```python
from build123d import *

# Parameters (mm, degrees)
BASE_W                 = 11.6
BASE_H                 = 22.8
MAIN_DEPTH             = 5
GEAR_AXIS_HOLES_D      = 5
M2_5_CLEARANCE_HOLE1_D = 2.9
FILLET1_R              = 3
FILLET2_R              = 1.5


with BuildPart() as part:
    # Base → Main (new body)
    with BuildSketch(Plane.XY):
        Polygon((0, 27.5), (-26.7, 27.5), (-26.7, -27.5), (0, -27.5), (0, -39.47), (26.6, -39.47), (31.6, -39.47), (31.6, 27.5), (26.6, 27.5), align=None)
        with Locations((13.3, -14.97)):
            Rectangle(BASE_W, BASE_H, mode=Mode.SUBTRACT)
    extrude(amount=MAIN_DEPTH)

    # Gear Axis Holes (through all)
    with Locations(Plane(origin=(0, 0, 0), x_dir=(-1, 0, 0), z_dir=(0, 0, -1))):
        with Locations((16.7, -20), (16.7, 20)):
            Hole(GEAR_AXIS_HOLES_D / 2)

    # M2.5 Clearance Hole1 (through all)
    with Locations(Plane.XY.offset(5)):
        with Locations((13.3, -0.47), (13.3, -29.47)):
            Hole(M2_5_CLEARANCE_HOLE1_D / 2)

    # Fillet1
    fillet1_edges = [part.edges().sort_by_distance(p)[0] for p in [
        (31.6, 27.5, 2.5),
        (31.6, -39.47, 2.5),
        (0, -39.47, 2.5),
        (0, -27.5, 2.5),
        (-26.7, -27.5, 2.5),
        (-26.7, 27.5, 2.5),
    ]]
    fillet(fillet1_edges, radius=FILLET1_R)

    # Fillet2
    fillet2_edges = [part.edges().sort_by_distance(p)[0] for p in [
        (19.1, -26.37, 2.5),
        (19.1, -3.57, 2.5),
        (7.5, -3.57, 2.5),
        (7.5, -26.37, 2.5),
    ]]
    fillet(fillet2_edges, radius=FILLET2_R)


solid = part.part
```
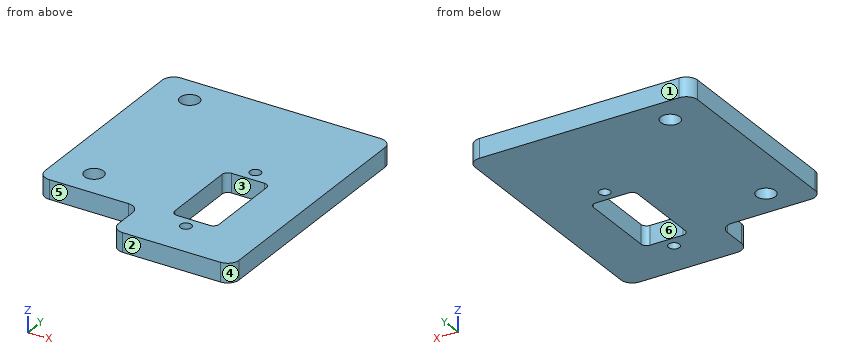
Geometry check sheet. Reference: the model listing, model coordinates, mm. Face numbers are marked on the shaded views. A direction names the side the tool comes from. Give positions to 0.01 mm unless a question says otherwise; leave off trailing zeros. Order: outer loops, then holes, each group sorted by start corner. A loop starts at its lowest first (then second) coordinate and runs counter-clockwise, first axis right, second up. Notation, with made-up numbers: (-24.75, 11) - (-2.75, 11) arc R15 cw to (-2.75, 32) - close; hole circle Ø8 at (62.25, 9.5). An arc over 180 degrees is marked (long way). Write item = value, one per line. Start each with the question number.
1) Access from +Z, -Z, +X, -X, +Y, -Y to the whole of each face (thin tool, end or side, straight path). Record for the marked faces 4, 5 and 6.
2) Section check B-B (x = 13.3). Enter the section's corners in (y, z).
3) Section check C-C (z = 1.75). Enter the section's corners in (x, y).
4) Section check A-A (y = -0.47). Enter the section's corners in (x, z).
5) Section check D-D (x = -16.7). Enter the section's corners in (y, z).
6) Draft check along Y on the marked faces 1, 2 and 3. Enter one of: released by +Y, released by -Y, zero draft, split by the parting line, or undercut.
7) Scan lines: L1, parallel to Y at x = -16.7, z = 1.9; L2, parallel to Y at x = 13.3, z = 3.9; L3, parallel to X at y = -17, z = 3.7. Record each from-to range of solid material in increasing order.
8) Gauge pin test, flat ends, axial feed: pin 1 Ø5 at (x, y) = (-1, 8) entering from -Z; pin 2 Ø4.5 at (x, y) = (-16.7, -20) entering from +Z; pin 3 Ø2.5 at (y, z) = (-33.5, 2) entering from -X; pin 4 Ø1.5 at (x, z) = (-13.5, 3) entering from -Y. Record the tip position at first contact, or that the pin passes through.
Geometry check:
q1.face_4 = +Z, -Z, +X, -Y
q1.face_5 = +Z, -Z, -X, -Y
q1.face_6 = +Z, -Z
q2.outline = (-39.47, 0) - (-30.92, 0) - (-30.92, 5) - (-39.47, 5) - close; (-28.02, 0) - (-26.37, 0) - (-26.37, 5) - (-28.02, 5) - close; (-3.57, 0) - (-1.92, 0) - (-1.92, 5) - (-3.57, 5) - close; (0.98, 0) - (27.5, 0) - (27.5, 5) - (0.98, 5) - close
q3.outline = (-26.7, -24.5) arc R3 ccw to (-23.7, -27.5) - (-3, -27.5) arc R3 cw to (0, -30.5) - (0, -36.47) arc R3 ccw to (3, -39.47) - (28.6, -39.47) arc R3 ccw to (31.6, -36.47) - (31.6, 24.5) arc R3 ccw to (28.6, 27.5) - (-23.7, 27.5) arc R3 ccw to (-26.7, 24.5) - close; hole circle Ø5 at (-16.7, -20); hole circle Ø5 at (-16.7, 20); hole (7.5, -24.87) arc R1.5 ccw to (9, -26.37) - (17.6, -26.37) arc R1.5 ccw to (19.1, -24.87) - (19.1, -5.07) arc R1.5 ccw to (17.6, -3.57) - (9, -3.57) arc R1.5 ccw to (7.5, -5.07) - close; hole circle Ø2.9 at (13.3, -29.47); hole circle Ø2.9 at (13.3, -0.47)
q4.outline = (-26.7, 0) - (11.85, 0) - (11.85, 5) - (-26.7, 5) - close; (14.75, 0) - (31.6, 0) - (31.6, 5) - (14.75, 5) - close
q5.outline = (-27.5, 0) - (-22.5, 0) - (-22.5, 5) - (-27.5, 5) - close; (-17.5, 0) - (17.5, 0) - (17.5, 5) - (-17.5, 5) - close; (22.5, 0) - (27.5, 0) - (27.5, 5) - (22.5, 5) - close
q6.face_1 = released by +Y
q6.face_2 = released by -Y
q6.face_3 = undercut
q7.L1 = -27.5 to -22.5, -17.5 to 17.5, 22.5 to 27.5
q7.L2 = -39.47 to -30.92, -28.02 to -26.37, -3.57 to -1.92, 0.98 to 27.5
q7.L3 = -26.7 to 7.5, 19.1 to 31.6
q8.pin_1 = 0
q8.pin_2 = through
q8.pin_3 = 0
q8.pin_4 = -27.5
